Work out the finished part from the listing and answer in its coordinate system (mm). A direction names the side the tool comes from. Give positions to 0.01 mm unless a question says otherwise; leave off trailing zeros. Order: outer loops, then holes, each group sorted by start corner. A loop starts at its lowest first (then second) coordinate and runs counter-clockwise, first axis right, second up. Notation, with made-up numbers: (-39.75, 40) -> (-23.75, 40) arc R19 cw to (-23.75, 47) -> close; hole circle Ø6 at (72.25, -32). An arc over 180 degrees is marked (long way). Answer as CSV lines item,"result". Start each with the question number.
1. Flat-ended cylindrical pins translate along their axes: pin 1 (4 mm diameter, centred on x = 93.5, z = 79, fed in from -Y); pin 2 (2 mm diameter, centred on x = 42.5, y = 68, fed in from -Z); pin 3 (8 mm diameter, centred on x = 14.5, z = 18, fed in from +Y). Find the tip coordinate at first contact, or state that the pin passes through.
2. For a pull along X with two mould halves and no side action, classify faces 4 (the flat face through (-56, 392, 90)), 5 (the cylindrical face through (9.764, 261.638, -1.26)), 6 (the cylindrical face through (30.04, 59.16, 95.38)) as released by +X, released by -X, zero draft, split by the parting line, or undercut.
3. A cutting plane is placed at C-C (z = 0). Give the vertices of the cut face in (x, y).
4. A cutting plane is placed at A-A (y = 336). Give the vertices of the cut face in (x, z), then the cut area to 3 significant figures.
5. For faces 1 (the flat face through (-110, 200, 1)), 2 (the flat face through (73, 120, 69)), 3 (the flat face through (110, 200, 1)), determine the directions among +Z, -Z, +X, -X, +Y, -Y from which every point of the face is accessible in a straight line to the end or side of a thin tool.
6. A cutting plane is placed at B-B (x = 0). Give the vertices of the cut face in (y, z).
7. A cutting plane is placed at D-D (z = 73). Give the vertices of the cut face in (x, y).
8. Find the intervals of material crossed by L1, parallel to X at y = 336, z = -32; L2, parallel to Y at x = 0, z = -11; L3, parallel to Y at x = -14.5, z = -137.5, in increasing order.
from build123d import *

# Parameters (mm, degrees)
SKETCH1_R                = 100
BOSS_EXTRUDE1_DEPTH      = 120
SKETCH2_R                = 160
BOSS_EXTRUDE2_DEPTH      = 16
SKETCH3_R                = 130
SKETCH3_R_2              = 75
BOSS_EXTRUDE3_DEPTH      = 90
BOSS_EXTRUDE4_REACH      = 402.125
BOSS_EXTRUDE4_END_RADIUS = 130
SKETCH4_W                = 220
SKETCH4_H                = 160


with BuildPart() as part:
    # Sketch1 → Boss-Extrude1 (new body)
    with BuildSketch(Plane(origin=(0, 0, 0), x_dir=(1, 0, 0), z_dir=(0, 1, 0))):
        with Locations(Location((0, 0, 0), (0, 0, 270))):
            Circle(SKETCH1_R)
    extrude(amount=BOSS_EXTRUDE1_DEPTH)

    # Sketch2 → Boss-Extrude2 (add)
    with BuildSketch(Plane(origin=(0, 120, 0), x_dir=(1, 0, 0), z_dir=(0, 1, 0))):
        with Locations(Location((0, 0, 0), (0, 0, 270))):
            Circle(SKETCH2_R)
    extrude(amount=BOSS_EXTRUDE2_DEPTH)



with BuildPart() as body_2:
    # Sketch3 → Boss-Extrude3 (new, symmetric)
    with BuildSketch(Plane.XY):
        with Locations(Location((0, 336, 0), (0, 0, 180))):
            Circle(SKETCH3_R)
        with Locations(Location((0, 336, 0), (0, 0, 180))):
            Circle(SKETCH3_R_2, mode=Mode.SUBTRACT)
    extrude(amount=BOSS_EXTRUDE3_DEPTH, both=True)


with BuildPart() as part_1:
    add(part.part)

    add(body_2.part)  # Boss-Extrude4 merges body 2
    # Boss-Extrude4: up to this cylinder (the profile starts outside it)
    boss_extrude4_end = Plane(origin=(0, 336, 0), z_dir=(0, 0, -1)) * Cylinder(BOSS_EXTRUDE4_END_RADIUS, 1065.25, mode=Mode.PRIVATE)
    # Sketch4 → Boss-Extrude4 (add, up to the surface)
    with BuildSketch(Plane(origin=(0, 136, 0), x_dir=(1, 0, 0), z_dir=(0, 1, 0)), mode=Mode.PRIVATE) as boss_extrude4_sk1:
        Rectangle(SKETCH4_W, SKETCH4_H)
    boss_extrude4_tool1 = extrude(boss_extrude4_sk1.sketch, amount=BOSS_EXTRUDE4_REACH, mode=Mode.PRIVATE) - boss_extrude4_end
    add(boss_extrude4_tool1.solids().sort_by_distance((0, 136, 0))[0])


solid = part_1.part
Answer sheet:
1,pin 1,"stops at y = 120"
1,pin 2,"stops at z = -90.98"
1,pin 3,"stops at y = 465.58"
2,face 4,"zero draft"
2,face 5,"undercut"
2,face 6,"split by the parting line"
3,outline,"(-160, 120) -> (-100, 120) -> (-100, 0) -> (100, 0) -> (100, 120) -> (160, 120) -> (160, 136) -> (110, 136) -> (110, 266.72) arc R130 ccw (long way) to (-110, 266.72) -> (-110, 136) -> (-160, 136) -> close; hole circle Ø150 at (0, 336)"
4,outline,"(-130, -90) -> (-75, -90) -> (-75, 90) -> (-130, 90) -> close; (75, -90) -> (130, -90) -> (130, 90) -> (75, 90) -> close"
4,area,"19,800 mm^2"
5,face 1,"+Z, -Z, -X"
5,face 2,"-Y"
5,face 3,"+Z, -Z, +X"
6,outline,"(0, -100) -> (120, -100) -> (120, -160) -> (136, -160) -> (136, -80) -> (206, -80) -> (206, -90) -> (261, -90) -> (261, 90) -> (206, 90) -> (206, 80) -> (136, 80) -> (136, 160) -> (120, 160) -> (120, 100) -> (0, 100) -> close; (411, -90) -> (466, -90) -> (466, 90) -> (411, 90) -> close"
7,outline,"(-142.38, 120) -> (-68.34, 120) -> (-68.34, 0) -> (68.34, 0) -> (68.34, 120) -> (142.38, 120) -> (142.38, 136) -> (110, 136) -> (110, 266.72) arc R130 ccw (long way) to (-110, 266.72) -> (-110, 136) -> (-142.38, 136) -> close; hole circle Ø150 at (0, 336)"
8,L1,"x = -130 to -75, 75 to 130"
8,L2,"y = 0 to 261, 411 to 466"
8,L3,"y = 120 to 136"
